Verification items for this drawing (mm, ordinates from the low corner). A direction names the side the tool comes from. Give positions to 0.01 mm unless a question says otherwise; leave off trailing zeros. Write each loop counter-clockwise with the first axis right and the second up, starting at its lowest first coordinate (ties: lowest second). Pieces come first, ordered by that corner, then holes. Notation, with made-up numbers: (-9, -32) -> (30, -32) arc R29 cw to (30, 5) -> close; hole circle Ø5 at (12.5, 26). An arc over 180 degrees is marked (long way). Use one line per item in the form item = value. Start each with the question number.
(1) Section check C-C, the plane x = 13.5. Record the cut outline in (y, z).
(2) Section check B-B, the plane y = 4.6. Record the cut outline in (x, z), plus the area to 3 significant figures.
(3) Release check for a two-part mould opening along Z. For the marked faces 6, 7, 8 and 9 record: pulls with the +Z half, pulls with the -Z half, needs draft (parallel to the pull), parting line crosses it, or undercut.
(4) Section check A-A, the plane z = 3.5. Record the cut outline in (x, y), plus the area to 4 significant figures.
(5) Scan lines: L1, parallel to X at y = 5.3, z = 14; L2, parallel to Z at x = 6.75, y = 4.15; L3, parallel to Z at x = 6.5, y = 2.9. Record each from-to range of solid material in increasing order.
(6) Depth check by flat-ended pin: pin 1 Ø4 at (x, z) = (2.5, 14) entering from -Y; pin 2 Ø3.5 at (x, y) = (8.5, 1) entering from +Z; pin 3 Ø3 at (x, z) = (13.5, 14) entering from +Y; pin 4 Ø3 at (x, z) = (12, 3) entering from +Y. Enter the tip coordinate at first touch or a pass-through.
(7) Section check D-D, the plane z = 14. Record the cut outline in (x, y).
(8) Set-up check for the marked faces 1, 2, 3, 4 and 5: record each of +Z, -Z, +X, -X, +Y, -Y from which the full face is reachable in a straight line by a thin tool's end or side.
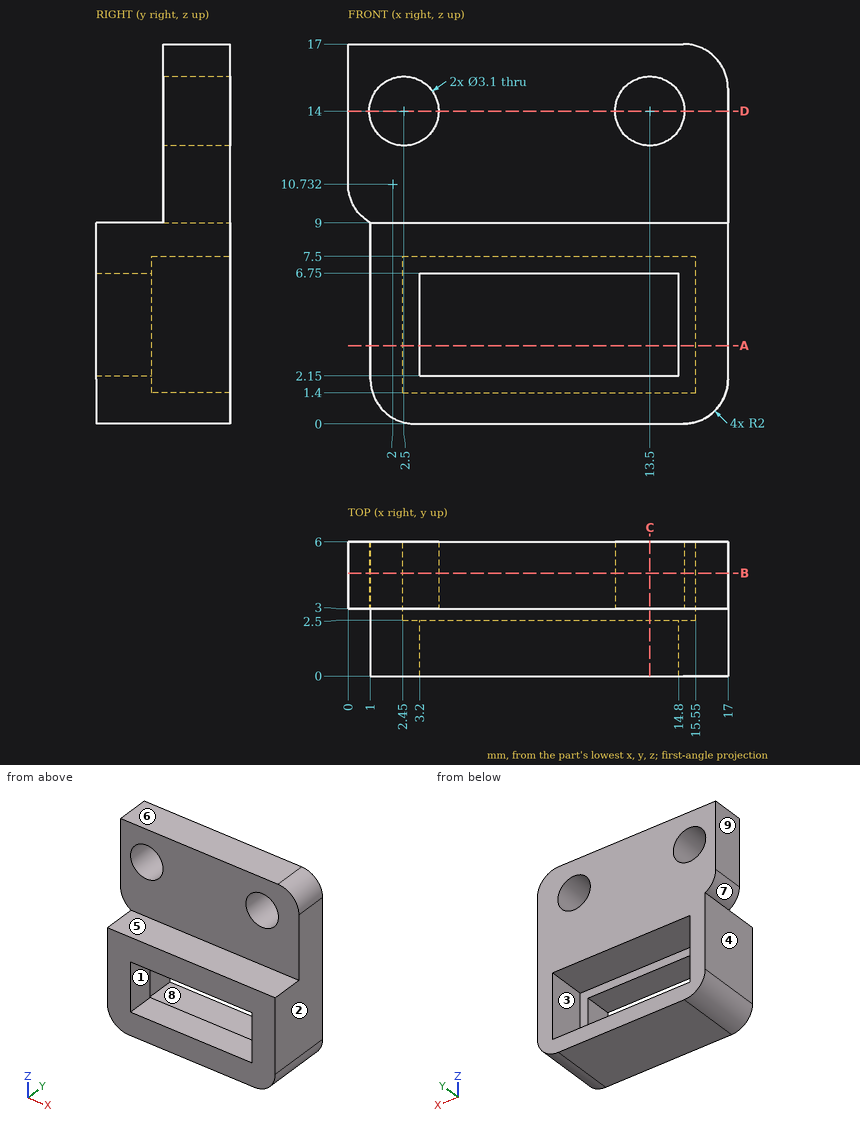
Completed:
q1.outline = (0, 0) -> (6, 0) -> (6, 1.4) -> (2.5, 1.4) -> (2.5, 2.15) -> (0, 2.15) -> close; (0, 6.75) -> (2.5, 6.75) -> (2.5, 7.5) -> (6, 7.5) -> (6, 12.45) -> (3, 12.45) -> (3, 9) -> (0, 9) -> close; (3, 15.55) -> (6, 15.55) -> (6, 17) -> (3, 17) -> close
q2.outline = (0, 10.73) arc R2 ccw to (1, 9) -> (1, 2) arc R2 ccw to (3, 0) -> (15, 0) arc R2 ccw to (17, 2) -> (17, 15) arc R2 ccw to (15, 17) -> (0, 17) -> close; hole circle Ø3.1 at (2.5, 14); hole (2.45, 1.4) -> (15.55, 1.4) -> (15.55, 7.5) -> (2.45, 7.5) -> close; hole circle Ø3.1 at (13.5, 14)
q2.area = 182 mm²
q3.face_6 = pulls with the +Z half
q3.face_7 = pulls with the -Z half
q3.face_8 = undercut
q3.face_9 = needs draft
q4.outline = (1, 0) -> (3.2, 0) -> (3.2, 2.5) -> (2.45, 2.5) -> (2.45, 6) -> (1, 6) -> close; (14.8, 0) -> (17, 0) -> (17, 6) -> (15.55, 6) -> (15.55, 2.5) -> (14.8, 2.5) -> close
q4.area = 21.15 mm²
q5.L1 = 0 to 0.95, 4.05 to 11.95, 15.05 to 17
q5.L2 = 0 to 1.4, 7.5 to 17
q5.L3 = 0 to 1.4, 7.5 to 9
q6.pin_1 = 3
q6.pin_2 = 9
q6.pin_3 = through
q6.pin_4 = 2.5
q7.outline = (0, 3) -> (0.95, 3) -> (0.95, 6) -> (0, 6) -> close; (4.05, 3) -> (11.95, 3) -> (11.95, 6) -> (4.05, 6) -> close; (15.05, 3) -> (17, 3) -> (17, 6) -> (15.05, 6) -> close
q8.face_1 = +Y, -Y
q8.face_2 = +Z, -Z, +X, +Y, -Y
q8.face_3 = +Y
q8.face_4 = -Z, -X, +Y, -Y
q8.face_5 = +Z, +X, -X, -Y
